Work out the finished part from the listing and answer in its coordinate system (mm). Face numbers are marked on the shaded views. Give positions to 0.01 mm unless a question says otherwise; leave off trailing zeros. Loops run counter-clockwise (first coordinate to the right, second up) from the corner with the lowest first, then second, coordinate; pieces in that order, holes last. Notation, with made-up numbers: (44.25, -4.75) - (53.25, -4.75) arc R18 cw to (53.25, 9.25) - close; hole circle Ø9 at (67.5, -10). An arc over 180 degrees is marked (long way). One line per question, with ' | ' between items. Start each with the question number.
1. Section D-D (y = 8) is taken. Determine the outline of the cut face in (x, z).
2. Section B-B (x = 10.25) is taken. Determine the outline of the cut face in (y, z).
3. Section A-A (z = 0) is taken. Determine the outline of the cut face in (x, y).
4. Find the intervals of material crossed by line 1 (X direction, y = 8.25, z = 0); line 2 (X direction, y = -0.25, z = -0.25), in increasing order.
5. Each of these flat-tipped pins is pushed along its axis until it touches: pin 1 (3.5 mm diameter, centred on x = 7, y = -2, fed in from +Z); pin 2 (12 mm diameter, centred on x = 5, z = 2, fed in from +Y); pin 3 (0.9 mm diameter, centred on y = -1, z = -1, fed in from +X). Where does it stop, or does it pass through?
6. For a pull along Z with two mould halves and no side action, classify the marked faces 1, 2 and 3 as released by +Z, released by -Z, zero draft, split by the parting line, or undercut.
7. Section C-C (x = 0) is taken. Determine the outline of the cut face in (y, z).
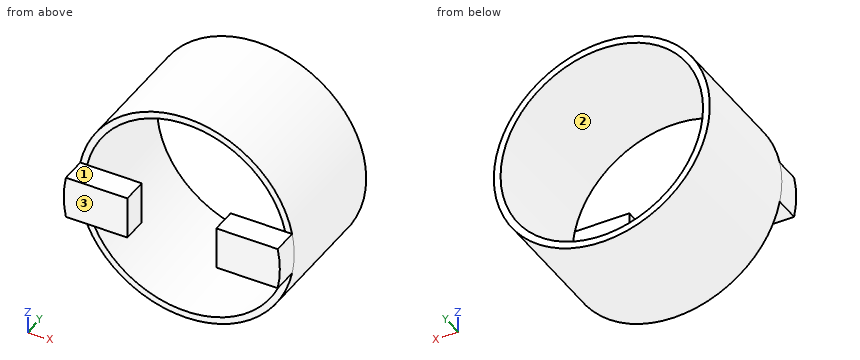
from build123d import *

# Parameters (mm, degrees)
SKETCH2_R           = 12.75
SKETCH2_R_2         = 11.95
BOSS_EXTRUDE1_DEPTH = 15
BOSS_EXTRUDE2_DEPTH = 3


with BuildPart() as part:
    # Sketch2 → Boss-Extrude1 (new body)
    with BuildSketch(Plane(origin=(0, 0, 0), x_dir=(1, 0, 0), z_dir=(0, 1, 0))):
        Circle(SKETCH2_R)
        Circle(SKETCH2_R_2, mode=Mode.SUBTRACT)
    extrude(amount=BOSS_EXTRUDE1_DEPTH)

    # Sketch3 → Boss-Extrude2 (add)
    with BuildSketch(Plane.XZ):
        with BuildLine():
            Line((5.25, -2.5), (5.25, 2.5))
            Line((5.25, 2.5), (12.5025, 2.5))
            ThreePointArc((12.5025, 2.5), (12.75, 0), (12.5025, -2.5))
            Line((12.5025, -2.5), (5.25, -2.5))
        make_face()
        with BuildLine():
            Line((-5.25, -2.5), (-12.5025, -2.5))
            ThreePointArc((-12.5025, -2.5), (-12.75, 0), (-12.5025, 2.5))
            Line((-12.5025, 2.5), (-5.25, 2.5))
            Line((-5.25, 2.5), (-5.25, -2.5))
        make_face()
    extrude(amount=BOSS_EXTRUDE2_DEPTH)


solid = part.part
Conclusion:
1) outline: circle Ø25.5 at (0, 0); hole circle Ø23.9 at (0, 0)
2) outline: (-3, -2.5) - (0, -2.5) - (0, 2.5) - (-3, 2.5) - close; (0, -7.58) - (15, -7.58) - (15, -6.14) - (0, -6.14) - close; (0, 6.14) - (15, 6.14) - (15, 7.58) - (0, 7.58) - close
3) outline: (-12.75, -3) - (-5.25, -3) - (-5.25, 0) - (-11.95, 0) - (-11.95, 15) - (-12.75, 15) - close; (5.25, -3) - (12.75, -3) - (12.75, 15) - (11.95, 15) - (11.95, 0) - (5.25, 0) - close
4) line 1: -12.75 to -11.95, 11.95 to 12.75 | line 2: -12.75 to -5.25, 5.25 to 12.75
5) pin 1: z = 2.5 | pin 2: y = 0 | pin 3: x = 12.74
6) face 1: released by +Z | face 2: undercut | face 3: zero draft
7) outline: (0, -12.75) - (15, -12.75) - (15, -11.95) - (0, -11.95) - close; (0, 11.95) - (15, 11.95) - (15, 12.75) - (0, 12.75) - close
